Autodesk Inventor part; units mm, degrees
ref_plane "YZ Plane" through (0, 0, 0) normal (1, 0, 0) x (0, 1, 0)
ref_plane "XZ Plane" through (0, 0, 0) normal (0, 1, 0) x (-1, 0, 0)
ref_plane "XY Plane" through (0, 0, 0) normal (0, 0, 1) x (1, 0, 0)
sketch "Sketch1" plane through (0, 0, 0) normal (1, 0, 0) x (0, 1, 0)
  circle A0 centre (0, 0) radius 30.48
  circle A1 centre (0, 0) radius 9.525
  circle A2 centre (25.3286, -1.9038) radius 3
  circle A3 centre (-25.3286, 1.9038) radius 3
  circle A4 centre (0, -33.0962) radius 11.43
  line L0 (27.3765, 13.4) -> (-27.3765, 13.4)
  line L1 (-25.3286, 1.9038) -> (25.3286, -1.9038) construction
  line L2 (0, -33.0962) -> (-25.3286, -33.0962)
  point P0 (10.5127, -28.6097)
  point P1 (-10.5127, -28.6097)
  dimension "d0" = 6
  dimension "d2" = 19.05
  dimension "d3" = 60.96
  dimension "d6" = 22.86
  dimension "d8" = 50.8
  dimension "d9" = 13.4
  dimension "d11" = 70
  dimension "d12" = 33.0962
extrude "Plate1" add sketch "Sketch1" along normal blind 3 contours A0 A4 L0
equation "\"BendRadius\" = Thickness"
equation "\"BendReliefWidth\" = Thickness"
equation "\"BendReliefDepth\" = 0.5 * Thickness"
equation "\"CornerReliefSize\" = 4 * Thickness"
equation "\"MinimumRemnant\" = 2 * Thickness"
equation "\"TransitionRadius\" = BendRadius"
equation "\"JacobiRadiusSize\" = BendRadius"
equation "\"GapSize\" = Thickness"
equation "\"d7\" = BendRadius"
properties part number "MotorSpacer" material "ABS Plastic"
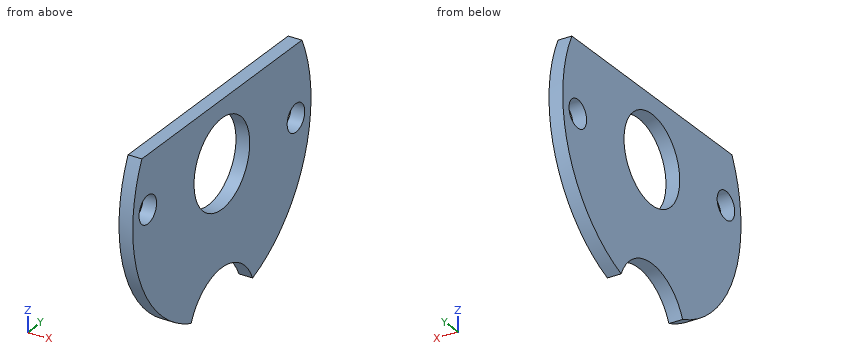
The listing builds one solid part. Answer for the finished solid, in the listing's coordinates (mm). Coordinates: 2 decimals unless noted, no trailing zeros. Write each loop counter-clockwise with the first axis right and the second up, starting at its lowest first coordinate (ties: lowest second). Pieces come first, ordered by that corner, then holes. Notation, with made-up numbers: (82.5, -5.5) -> (94.5, -5.5) arc R5 cw to (94.5, -0.5) -> close; hole circle Ø11 at (1.25, 64). An arc over 180 degrees is marked (long way). Write each question's results on one line, items separated by ' | '. Start each with the question number.
1) A cutting plane is placed at A-A (y = 0). Determine the outline of the cut face in (x, z) (3 decimals).
2) Straight lines are drawn through the part: probe 1 along Y at (x, z) = (2.7, 2); probe 2 along Y at (x, z) = (0.2, -2.5); probe 3 along Y at (x, z) = (0.2, -23.5). For each, find the intervals that lie inside material, in ascending order.
3) Flat-ended cylindrical pins translate along their axes: pin 1 Ø5 at (y, z) = (25.33, -1.9) entering from -X; pin 2 Ø1.5 at (x, z) = (2, -15.5) entering from +Y. Find the tip coordinate at first contact, or state that the pin passes through.
4) A cutting plane is placed at D-D (y = -6.5). Determine the outline of the cut face in (x, z), then the cut area to 3 significant figures.
5) A cutting plane is placed at B-B (z = 0). Determine the outline of the cut face in (x, y) (3 decimals), then the cut area to 3 significant figures.
6) A cutting plane is placed at C-C (x = 1.9). Count the separate pieces of the cut face and the enclosed holes in it, then the cut area to 3 significant figures.
Values follow:
1) outline: (0, -21.666) -> (3, -21.666) -> (3, -9.525) -> (0, -9.525) -> close; (0, 9.525) -> (3, 9.525) -> (3, 13.4) -> (0, 13.4) -> close
2) probe 1: -30.41 to -28.33, -22.33 to -9.31, 9.31 to 30.41 | probe 2: -30.38 to -9.19, 9.19 to 22.39, 28.27 to 30.38 | probe 3: -19.41 to -6.21, 6.21 to 19.41
3) pin 1: through | pin 2: y = 26.67
4) outline: (0, -23.69) -> (3, -23.69) -> (3, -6.96) -> (0, -6.96) -> close; (0, 6.96) -> (3, 6.96) -> (3, 13.4) -> (0, 13.4) -> close | area: 69.5 mm²
5) outline: (0, -30.48) -> (3, -30.48) -> (3, -27.647) -> (0, -27.647) -> close; (0, -23.01) -> (3, -23.01) -> (3, -9.525) -> (0, -9.525) -> close; (0, 9.525) -> (3, 9.525) -> (3, 23.01) -> (0, 23.01) -> close; (0, 27.647) -> (3, 27.647) -> (3, 30.48) -> (0, 30.48) -> close | area: 97.9 mm²
6) separate pieces: 1 | enclosed holes: 3 | area: 1,780 mm²
